Source: CAD feature listing. Evaluate the final solid. Frame: model axes, mm. A direction names the side the tool comes from. Coordinates: 2 decimals unless noted, no trailing zeros. Loops run counter-clockwise (first coordinate to the right, second up) from the corner with the lowest first, then second, coordinate; pieces in that order, holes last.
```python
from build123d import *

# Parameters (mm, degrees)
D_RA1_D         = 3.5
D_RA1_DEPTH     = 4
D_RA1_TIP       = 1.051506083
VYSUNOUT1_REACH = 11.055


with BuildPart() as part:
    # Skica1 → Otočit kolem osy1 (revolve)
    with BuildSketch(Plane(origin=(0, 0, 0), x_dir=(1, 0, 0), z_dir=(0, 1, 0))):
        Polygon((0, 0), (0, 2.5), (0.5, 3), (7, 3), (8, 2.422649731), (8, 0), align=None)
    revolve(axis=Axis((8, 0, 0), (-1, 0, 0)))

    # Díra1
    with Locations(Plane.ZY):
        with Locations((0, 0)):
            Hole(D_RA1_D / 2, depth=D_RA1_DEPTH)
            with Locations((0, 0, -(D_RA1_DEPTH + D_RA1_TIP / 2))):  # 118° drill point
                Cone(0, D_RA1_D / 2, D_RA1_TIP, mode=Mode.SUBTRACT)

    # Vysunout1: up to this cone (the profile starts inside it)
    vysunout1_end = Plane(origin=(0, 0, 0), z_dir=(-1, 0, 0)).offset(-5.051505083) * Cone(1.664e-06, 41.629661224, 25.013623013, align=(Align.CENTER, Align.CENTER, Align.MIN), mode=Mode.PRIVATE)
    # Skica4 → Vysunout1 (add, up to the surface)
    with BuildSketch(Plane.ZY, mode=Mode.PRIVATE) as vysunout1_sk1:
        with BuildLine():
            Line((-1.75, 0), (-0.875, 1.515544457))
            ThreePointArc((-0.875, 1.515544457), (-1.515544457, 0.875), (-1.75, 0))
        make_face()
    vysunout1_tool1 = extrude(vysunout1_sk1.sketch, amount=-VYSUNOUT1_REACH, mode=Mode.PRIVATE) & vysunout1_end
    add(vysunout1_tool1.solids().sort_by_distance((0, 0.804943, -1.394203))[0])
    # Skica4 → Vysunout1 (add, up to the surface)
    with BuildSketch(Plane.ZY, mode=Mode.PRIVATE) as vysunout1_sk2:
        with BuildLine():
            ThreePointArc((0.875, 1.515544457), (0, 1.75), (-0.875, 1.515544457))
            Line((-0.875, 1.515544457), (0.875, 1.515544457))
        make_face()
    vysunout1_tool2 = extrude(vysunout1_sk2.sketch, amount=-VYSUNOUT1_REACH, mode=Mode.PRIVATE) & vysunout1_end
    add(vysunout1_tool2.solids().sort_by_distance((0, 1.609887, 0))[0])
    # Skica4 → Vysunout1 (add, up to the surface)
    with BuildSketch(Plane.ZY, mode=Mode.PRIVATE) as vysunout1_sk3:
        with BuildLine():
            ThreePointArc((1.75, 0), (1.515544457, 0.875), (0.875, 1.515544457))
            Line((0.875, 1.515544457), (1.75, 0))
        make_face()
    vysunout1_tool3 = extrude(vysunout1_sk3.sketch, amount=-VYSUNOUT1_REACH, mode=Mode.PRIVATE) & vysunout1_end
    add(vysunout1_tool3.solids().sort_by_distance((0, 0.804943, 1.394203))[0])
    # Skica4 → Vysunout1 (add, up to the surface)
    with BuildSketch(Plane.ZY, mode=Mode.PRIVATE) as vysunout1_sk4:
        with BuildLine():
            ThreePointArc((0.875, -1.515544457), (1.515544457, -0.875), (1.75, 0))
            Line((1.75, 0), (0.875, -1.515544457))
        make_face()
    vysunout1_tool4 = extrude(vysunout1_sk4.sketch, amount=-VYSUNOUT1_REACH, mode=Mode.PRIVATE) & vysunout1_end
    add(vysunout1_tool4.solids().sort_by_distance((0, -0.804943, 1.394203))[0])
    # Skica4 → Vysunout1 (add, up to the surface)
    with BuildSketch(Plane.ZY, mode=Mode.PRIVATE) as vysunout1_sk5:
        with BuildLine():
            Line((0.875, -1.515544457), (-0.875, -1.515544457))
            ThreePointArc((-0.875, -1.515544457), (0, -1.75), (0.875, -1.515544457))
        make_face()
    vysunout1_tool5 = extrude(vysunout1_sk5.sketch, amount=-VYSUNOUT1_REACH, mode=Mode.PRIVATE) & vysunout1_end
    add(vysunout1_tool5.solids().sort_by_distance((0, -1.609887, 0))[0])
    # Skica4 → Vysunout1 (add, up to the surface)
    with BuildSketch(Plane.ZY, mode=Mode.PRIVATE) as vysunout1_sk6:
        with BuildLine():
            Line((-0.875, -1.515544457), (-1.75, 0))
            ThreePointArc((-1.75, 0), (-1.515544457, -0.875), (-0.875, -1.515544457))
        make_face()
    vysunout1_tool6 = extrude(vysunout1_sk6.sketch, amount=-VYSUNOUT1_REACH, mode=Mode.PRIVATE) & vysunout1_end
    add(vysunout1_tool6.solids().sort_by_distance((0, -0.804943, -1.394203))[0])

    # Skica5 → Odebrat otočením1 (revolve, cut)
    with BuildSketch(Plane(origin=(0, 0, 0), x_dir=(1, 0, 0), z_dir=(0, 1, 0))):
        Polygon((0, 1.75), (1.010362971, 0), (0, 0), align=None)
    revolve(axis=Axis((1.010362971, 0, 0), (-1, 0, 0)), mode=Mode.SUBTRACT)


solid = part.part
```
Q1. Material intervals for line 1 along Z through (x, y) = (2.75, -0.7); line 2 along Y through (x, z) = (2.5, -1.1); line 3 along Y through (x, z) = (3, -1.6), sorted ascending.
Q2. First-contact query: pin 1 Ø1.5 at (x, z) = (3.5, 1.5) entering from +Y; pin 2 Ø1.5 at (x, y) = (1, 1) entering from -Z; pin 3 Ø1 at (x, z) = (3, 2) entering from -Y. Flat tips, straight axial feed; report the tip coordinate or a pass-through.
Q3. Draft query along Y for faces 1 (the flat face through (8, 0, 0)), 2 (the flat face through (2.041, -0.747, 1.319)), 3 (the cylindrical face through (4, 0, 3)). Return one class per face: released by +Y, released by -Y, zero draft, split by the parting line, or undercut.
Q4. Section query A-A on x = 4.25. Return the cut outline in (y, z), then the cut area to 3 significant figures.
Q5. Reachability of faces 4 (the flat face through (0, 2, 1)), 5 (the flat face through (2.041, 0.747, -1.319)) from +Z, -Z, +X, -X, +Y, -Y: full face, straight path, thin tool, end or side. Return the list, or none.
Resolved:
1. line 1: z = -2.92 to -1.35, 1.35 to 2.92
1. line 2: y = -2.79 to -1.13, 1.13 to 2.79
1. line 3: y = -2.54 to -0.26, 0.26 to 2.54
2. pin 1: stops at y = 2.9
2. pin 2: stops at z = -2.99
2. pin 3: stops at y = -2.6
3. face 1: zero draft
3. face 2: undercut
3. face 3: split by the parting line
4. outline: circle Ø6 at (0, 0); hole circle Ø2.67 at (0, 0)
4. area: 22.7 mm2
5. face 4: +Z, -Z, -X, +Y, -Y
5. face 5: -X
